Could you check a few things on this model? Use its own coordinates, in mm. Face numbers are marked on the shaded views. A direction names the side the tool comes from. Coordinates: 2 decimals unless noted, no trailing zeros. Loops run counter-clockwise (first coordinate to the right, second up) from the corner with the lowest first, then second, coordinate; pieces in that order, holes last. Notation, with made-up numbers: (-11.75, -16.5) - (25.25, -16.5) arc R32 cw to (25.25, 11.5) - close; hole circle Ø11 at (36.25, -22). An arc over 180 degrees is marked (long way). One line per item, written item: value. Start each with the question number.
(1) If I drill on line 1 along X through (y, z) = (-3.5, -31); line 2 along X through (y, z) = (-6, 12.5); line 3 along Y through (x, z) = (11, -16.5), over which ranges is the centre line in solid material (lowest first)? Write a range as from..to.
(2) On a 3-axis mill with a long thin cutter (end or side, diameter ignored), from which of +Z, -Z, +X, -X, +Y, -Y can I reach the whole of each face in a straight line? I mean the marked faces 5, 6 and 7. Say none if no direction works.
(3) If we section it at A-A on y = 0: Write out the boundary of the cut face in (x, z), then the cut area to 3 significant figures.
(4) I'm going to push flat-ended pins straight in: P1, Ø1, axis at y = -15.5, z = 12.5, coming from the +X side; P2, Ø10, axis at y = -15.5, z = 2, coming from the -X side; P3, Ø3, axis at y = -19.5, z = 19.5, coming from the -X side. Where does each tip first touch, or does it pass through?
(5) If we section it at D-D on y = -19.5: Write out the boundary of the cut face in (x, z).
(6) If we section it at B-B on z = -30.5: Write out the boundary of the cut face in (x, y).
(7) If we mould it in two halves opening along X, with no side actions, what happens to the marked faces 1, 2, 3 and 4? For each: pulls with the +X half, pulls with the -X half, needs draft (parallel to the pull), parting line crosses it, or undercut.
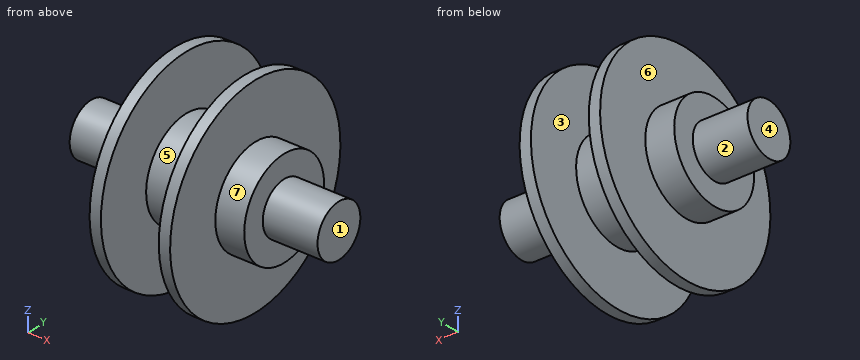
```python
from build123d import *


with BuildPart() as f1:
    # F0 (on Front) → F1 (revolve)
    with BuildSketch(Plane.XZ):
        Polygon((-42.7736, 0), (0, 0), (0, 16.8656), (-9.9822, 16.8656), (-9.9822, 35.941), (-13.8938, 35.941), (-13.8938, 16.8656), (-23.876, 16.8656), (-23.876, 9.0424), (-42.7736, 9.0424), align=None)
        Polygon((0, 16.8656), (0, 0), (42.7736, 0), (42.7736, 9.0424), (23.876, 9.0424), (23.876, 16.8656), (13.8938, 16.8656), (13.8938, 35.941), (9.9822, 35.941), (9.9822, 16.8656), align=None)
    revolve(axis=Axis((-21.3868, 0, 0), (1, 0, 0)))


solid = f1.part
```
Values:
1. line 1: x = -13.89..-9.98, 9.98..13.89
1. line 2: x = -23.88..23.88
1. line 3: y = -31.93..31.93
2. face 5: none
2. face 6: -X
2. face 7: +X
3. outline: (-42.77, -9.04) - (-23.88, -9.04) - (-23.88, -16.87) - (-13.89, -16.87) - (-13.89, -35.94) - (-9.98, -35.94) - (-9.98, -16.87) - (9.98, -16.87) - (9.98, -35.94) - (13.89, -35.94) - (13.89, -16.87) - (23.88, -16.87) - (23.88, -9.04) - (42.77, -9.04) - (42.77, 9.04) - (23.88, 9.04) - (23.88, 16.87) - (13.89, 16.87) - (13.89, 35.94) - (9.98, 35.94) - (9.98, 16.87) - (-9.98, 16.87) - (-9.98, 35.94) - (-13.89, 35.94) - (-13.89, 16.87) - (-23.88, 16.87) - (-23.88, 9.04) - (-42.77, 9.04) - close
3. area: 2,590 mm2
4. P1: stops at x = 13.89
4. P2: stops at x = -23.88
4. P3: stops at x = -13.89
5. outline: (-13.89, -30.19) - (-9.98, -30.19) - (-9.98, 30.19) - (-13.89, 30.19) - close; (9.98, -30.19) - (13.89, -30.19) - (13.89, 30.19) - (9.98, 30.19) - close
6. outline: (-13.89, -19.01) - (-9.98, -19.01) - (-9.98, 19.01) - (-13.89, 19.01) - close; (9.98, -19.01) - (13.89, -19.01) - (13.89, 19.01) - (9.98, 19.01) - close
7. face 1: pulls with the +X half
7. face 2: needs draft
7. face 3: undercut
7. face 4: pulls with the -X half
